from build123d import *

# Parameters (mm, degrees)
EXTRUDE_1_DEPTH     = 1
CUT_EXTRUDE_1_DEPTH = 35.313434576
SKETCH_5_R          = 1.5
CUT_EXTRUDE_2_DEPTH = 35.313434576
CUT_EXTRUDE1_DEPTH  = 1


with BuildPart() as part:
    # Эскиз1 → Бобышка-Вытянуть1 (new body)
    with BuildSketch(Plane(origin=(0, 0, 0), x_dir=(0, 0, -1), z_dir=(1, 0, 0))):
        Polygon((28.216339104, 4.507181273), (28.216339104, -19.5), (-28.216339104, -19.5), (-14.355786533, 4.507181273), align=None)
    extrude(amount=EXTRUDE_1_DEPTH)

    # Эскиз3 → Вырез-Вытянуть1 (cut, through all)
    with BuildSketch(Plane.ZY):
        with BuildLine():
            Line((-1.216339104, -7.8), (-11.216339104, -7.8))
            ThreePointArc((-11.216339104, -7.8), (-12.064867241, -8.151471863), (-12.416339104, -9))
            Line((-12.416339104, -9), (-12.416339104, -16.5))
            ThreePointArc((-12.416339104, -16.5), (-12.064867241, -17.348528137), (-11.216339104, -17.7))
            Line((-11.216339104, -17.7), (-1.216339104, -17.7))
            ThreePointArc((-1.216339104, -17.7), (-0.367810966, -17.348528137), (-0.016339104, -16.5))
            Line((-0.016339104, -16.5), (-0.016339104, -9))
            ThreePointArc((-0.016339104, -9), (-0.367810966, -8.151471863), (-1.216339104, -7.8))
        make_face()
    extrude(amount=-CUT_EXTRUDE_1_DEPTH, mode=Mode.SUBTRACT)

    # Эскиз5 → Вырез-Вытянуть2 (cut, through all)
    with BuildSketch(Plane.ZY):
        with Locations((-12.216339104, -2)):
            Circle(SKETCH_5_R)
        with Locations((-0.387535442, -2)):
            Circle(SKETCH_5_R)
    extrude(amount=-CUT_EXTRUDE_2_DEPTH, mode=Mode.SUBTRACT)

    # Sketch2 → Cut-Extrude1 (cut)
    with BuildSketch(Plane(origin=(1, 0, 0), x_dir=(0, 0, -1), z_dir=(1, 0, 0))):
        with BuildLine():
            Line((14.058648973, -4.786), (-2.125047218, -4.786))
            ThreePointArc((-2.125047218, -4.786), (-3.018111901, -5.192151072), (-3.309660896, -6.12891273))
            Line((-3.309660896, -6.12891273), (-3.309660896, -16.154222982))
            ThreePointArc((-3.309660896, -16.154222982), (-3.019412686, -17.092766498), (-2.125394323, -17.5))
            Line((-2.125394323, -17.5), (14.058301867, -17.5))
            ThreePointArc((14.058301867, -17.5), (14.95365068, -17.095122111), (15.246339104, -16.157087417))
            Line((15.246339104, -16.157087417), (15.246339104, -6.131777166))
            ThreePointArc((15.246339104, -6.131777166), (14.95495311, -5.191959061), (14.058648973, -4.786))
        make_face()
    extrude(amount=-CUT_EXTRUDE1_DEPTH, mode=Mode.SUBTRACT)


solid = part.part
Build history of the part. All positions in model axes, mm. A direction names the side the tool comes from. Give positions to 0.01 mm unless a question says otherwise; leave off trailing zeros. Loops run counter-clockwise (first coordinate to the right, second up) from the corner with the lowest first, then second, coordinate; pieces in that order, holes last. Notation, with made-up numbers: (24, 20.25) - (35, 20.25) arc R33 ccw to (35, 54.25) - close; hole circle Ø10 at (24.25, 39.5). An arc over 180 degrees is marked (long way). Write item = value, one per line. Start each with the question number.
1) Band-saw the part on A-A on z = -8.5. Give the cut face in (x, y).
2) Drop flat-ended pins along their axis: pin 1 Ø0.5 at (x, y) = (0.5, -10) entering from +Z; pin 2 Ø2.5 at (y, z) = (-2, -12.22) entering from -X. Give the stop position or say it passes through.
3) Band-saw the part on B-B on x = 0.65. Give the cut face in (y, z), plus the area to 3 significant figures.
4) Band-saw the part on C-C on y = -16.75. Give the cut face in (x, z), plus the area to 3 significant figures.
5) Probe probe 1 along Y at (x, z) = (0.7, -4); probe 2 along Z at (x, y) = (0.4, -3.25); probe 3 along Z at (x, y) = (0.75, -1). List the from-to ranges inside material, lowest first. Write a range as from..to.
6) Pull direction Z, two halves, no side cores. Call faces 3 (the flat face through (0.5, -7.3, -28.216)), 4 (the flat face through (0.49, -7.66, 21.38)), 5 (the flat face through (0.5, -17.5, -13)), 6 (the flat face through (1, -2, -7)): +Z half, -Z half, draft (parallel to the pull), parting line (faces both ways), or undercut.
7) Tool access for faces 1 (the flat face through (0.5, -19.5, -0.4)), 2 (the flat face through (0.5, -17.7, -6.3)): list every direction of +Z, -Z, +X, -X, +Y, -Y with a clear straight run to the whole face (end or side of a thin tool).
8) Band-saw the part on D-D on z = 0.5. Give the cut face in (x, y).
Final values:
q1.outline = (0, -19.5) - (1, -19.5) - (1, -17.7) - (0, -17.7) - close; (0, -4.79) - (1, -4.79) - (1, 4.51) - (0, 4.51) - close
q2.pin_1 = 22.88
q2.pin_2 = through
q3.outline = (-19.5, -28.22) - (4.51, -28.22) - (4.51, 14.36) - (-19.5, 28.22) - close; hole (-17.7, -11.22) arc R1.2 ccw to (-17.5, -11.88) - (-17.5, -14.06) arc R1.2 ccw to (-16.16, -15.25) - (-6.13, -15.25) arc R1.2 ccw to (-4.79, -14.06) - (-4.79, 2.13) arc R1.2 ccw to (-6.13, 3.31) - (-16.15, 3.31) arc R1.2 ccw to (-17.5, 2.13) - (-17.5, -0.55) arc R1.2 ccw to (-17.7, -1.22) - close; hole circle Ø3 at (-2, -12.22); hole circle Ø3 at (-2, -0.39)
q3.area = 937 mm²
q4.outline = (0, -28.22) - (1, -28.22) - (1, -15.17) - (0, -15.17) - close; (0, 3.23) - (1, 3.23) - (1, 26.63) - (0, 26.63) - close
q4.area = 36.4 mm²
q5.probe_1 = -19.5..-17.7, -4.79..4.51
q5.probe_2 = -28.22..-13.05, -11.39..-1.22, 0.44..18.83
q5.probe_3 = -28.22..-13.33, -11.1..-1.51, 0.73..17.54
q6.face_3 = -Z half
q6.face_4 = +Z half
q6.face_5 = undercut
q6.face_6 = draft
q7.face_1 = +Z, -Z, +X, -X, -Y
q7.face_2 = +X, -X
q8.outline = (0, -19.5) - (1, -19.5) - (1, -17.5) - (0, -17.5) - close; (0, -4.79) - (1, -4.79) - (1, -3.21) - (0, -3.21) - close; (0, -0.79) - (1, -0.79) - (1, 4.51) - (0, 4.51) - close
